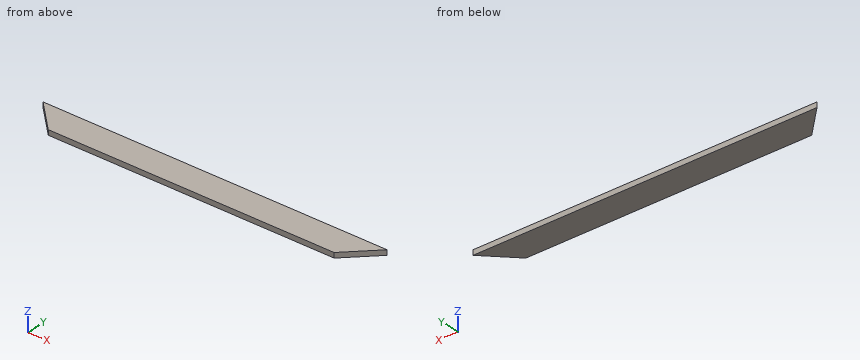
from build123d import *

# Parameters (mm, degrees)
F0_W     = 1420
F0_H     = 120
F1_DEPTH = 21
F2_SIZE  = 119.99999


# Not quite as in the source:
# - a fillet or chamfer is up to 0.001 mm smaller than in the source, because OpenCascade refuses the exact size


with BuildPart() as f1:
    # F0 (on Top) → F1 (new body)
    with BuildSketch(Plane.XY):
        Rectangle(F0_W, F0_H)
    extrude(amount=F1_DEPTH)

    # F2 (size 120 in the source; OpenCascade refuses exactly that, so slightly less here)
    f2_edges = [f1.edges().sort_by_distance(p)[0] for p in [
        (-710, -60, 10.5),
        (710, -60, 10.5),
    ]]
    chamfer(f2_edges, length=F2_SIZE)


solid = f1.part
Verification items for the finished model (mm, model axes). Coordinates: 2 decimals unless noted, no trailing zeros. Loops run counter-clockwise (first coordinate to the right, second up) from the corner with the lowest first, then second, coordinate; pieces in that order, holes last. Notation, with made-up numbers: (-14.5, 49) -> (22.5, 49) arc R12 ccw to (22.5, 69) -> close; hole circle Ø9 at (47, 13.25). An arc over 180 degrees is marked (long way). Write each question's results on one line, items separated by ' | '.
Item 1: Gauge pin test, flat ends, axial feed: pin 1 (2 mm diameter, centred on y = 44, z = 16, fed in from +X); pin 2 (1.5 mm diameter, centred on y = -11, z = 3.5, fed in from +X); pin 3 (4 mm diameter, centred on y = -3.5, z = 6, fed in from -X). Record the tip position at first contact, or that the pin passes through.
Found:
pin 1: stops at x = 695 | pin 2: stops at x = 639.75 | pin 3: stops at x = -648.5
Item 2: Section check C-C, the plane y = 34. Enter the section's corners in (x, z).
Found:
outline: (-684, 0) -> (684, 0) -> (684, 21) -> (-684, 21) -> close
Item 3: Material ranges on L1, parallel to X at y = 21.5, z = 6.5; L2, parallel to X at y = 53, z = 4.5; L3, parallel to Y at x = -639.5, z = 7, recorded low to high.
Found:
L1: x = -671.5 to 671.5 | L2: x = -703 to 703 | L3: y = -10.5 to 60
Item 4: Section check B-B, the plane y = -30. Enter the section's corners in (x, z).
Found:
outline: (-620, 0) -> (620, 0) -> (620, 21) -> (-620, 21) -> close
